from build123d import *

# Parameters (mm, degrees)
ESTRUSIONE_ESTRUSIONE1_DEPTH      = 2
ESTRUSIONE_ESTRUSIONE1_DEPTH_BACK = 2


with BuildPart() as part:
    # Forma aletta → Estrusione-Estrusione1 (new, two sides: drawn at the far end of the back side and taken through both)
    with BuildSketch(Plane(origin=(0, 0, 0), x_dir=(1, 0, 0), z_dir=(0, 1, 0)).offset(-ESTRUSIONE_ESTRUSIONE1_DEPTH_BACK)):
        Polygon((0, 300), (0, 50), (-10, 50), (-10, 0), (0, 0), (140, 0), (140, 150), align=None)
    extrude(amount=ESTRUSIONE_ESTRUSIONE1_DEPTH + ESTRUSIONE_ESTRUSIONE1_DEPTH_BACK)


solid = part.part
Could you check a few things on this model? Use its own coordinates, in mm. Give positions to 0.01 mm unless a question says otherwise; leave off trailing zeros. Order: outer loops, then holes, each group sorted by start corner. A loop starts at its lowest first (then second) coordinate and runs counter-clockwise, first axis right, second up. Notation, with made-up numbers: (46.5, 2.25) -> (55.5, 2.25) arc R12 ccw to (55.5, 7.25) -> close; hole circle Ø6 at (71, -28). An arc over 180 degrees is marked (long way). Return JSON: item names as keys, results as strings.
1. For pin 1 Ø1.2 at (y, z) = (0.5, -153.5) entering from -X, with a flat end and sliding along its axis, tell me the tip position at first contact or that it passes through.
Answer list:
{"pin 1": "stops at x = 0"}
2. Imagine slicing it at C-C on z = -244.5. List the corners of the cut face in (x, y) for me.
Answer list:
{"outline": "(0, -2) -> (51.8, -2) -> (51.8, 2) -> (0, 2) -> close"}
3. Imagine slicing it at B-B on x = 52.5. List the corners of the cut face in (y, z) for me, then the cut area to 3 significant figures.
Answer list:
{"outline": "(-2, -243.75) -> (2, -243.75) -> (2, 0) -> (-2, 0) -> close", "area": "975 mm2"}
4. I need wall thicknesses on line 1 (X direction, y = -1.2, z = -136.5); line 2 (Z direction, x = 79, y = -0.6); line 3 (Z direction, x = 89, y = 0.65). Which ranges of each line are inside material? Lowest first, please. Write a range as from..to.
Answer list:
{"line 1": "x = 0..140", "line 2": "z = -215.36..0", "line 3": "z = -204.64..0"}
5. Imagine slicing it at A-A on y = 1.4. List the corners of the cut face in (x, z) for me.
Answer list:
{"outline": "(-10, -50) -> (0, -50) -> (0, -300) -> (140, -150) -> (140, 0) -> (-10, 0) -> close"}
